```python
from build123d import *

# Parameters (mm, degrees)
SKETCH1_W            = 30
SKETCH1_H            = 70
BOSS_EXTRUDE1_DEPTH  = 1.57
M2_CLEARANCE_HOLE1_D = 2.4
CUT_EXTRUDE1_REACH   = 40.111
SKETCH6_R            = 0.55
LPATTERN1_COUNT      = 15
LPATTERN1_PITCH      = 2.54
SKETCH7_W            = 30
SKETCH7_H            = 20
CUT_EXTRUDE2_DEPTH   = 39.111217509
M2_CLEARANCE_HOLE2_D = 2.4


with BuildPart() as part:
    # Sketch1 → Boss-Extrude1 (new body)
    with BuildSketch(Plane(origin=(0, 0, 0), x_dir=(1, 0, 0), z_dir=(0, 1, 0))):
        Rectangle(SKETCH1_W, SKETCH1_H)
    extrude(amount=BOSS_EXTRUDE1_DEPTH)

    # M2 Clearance Hole1 (through all)
    with Locations(Plane(origin=(0, 1.57, 0), x_dir=(1, 0, 0), z_dir=(0, 1, 0))):
        with Locations((13, 33), (-13, 33), (-13, -33), (13, -33)):
            Hole(M2_CLEARANCE_HOLE1_D / 2)

    # Sketch6 → Cut-Extrude1 (cut, up to next)
    with BuildSketch(Plane(origin=(0, 1.57, 0), x_dir=(1, 0, 0), z_dir=(0, 1, 0)), mode=Mode.PRIVATE) as cut_extrude1_sk1:
        with Locations(Location((6.93, 18.93, 0), (0, 0, 270))):
            Circle(SKETCH6_R)
    cut_extrude1_tool1 = extrude(cut_extrude1_sk1.sketch, amount=-CUT_EXTRUDE1_REACH, mode=Mode.PRIVATE) & part.part
    # Sketch6 → Cut-Extrude1 (cut, up to next)
    with BuildSketch(Plane(origin=(0, 1.57, 0), x_dir=(1, 0, 0), z_dir=(0, 1, 0)), mode=Mode.PRIVATE) as cut_extrude1_sk2:
        with Locations(Location((-8.43, 18.93, 0), (0, 0, 270))):
            Circle(SKETCH6_R)
    cut_extrude1_tool2 = extrude(cut_extrude1_sk2.sketch, amount=-CUT_EXTRUDE1_REACH, mode=Mode.PRIVATE) & part.part
    cut_extrude1_1 = cut_extrude1_tool1.solids().sort_by_distance((6.93, 1.57, -18.93))[0]
    add(cut_extrude1_1, mode=Mode.SUBTRACT)
    cut_extrude1_2 = cut_extrude1_tool2.solids().sort_by_distance((-8.43, 1.57, -18.93))[0]
    add(cut_extrude1_2, mode=Mode.SUBTRACT)
    cut_extrude1 = cut_extrude1_1 + cut_extrude1_2  # Cut-Extrude1 as one shape, for the pattern or mirror that repeats it

    # LPattern1: Cut-Extrude1 ×15
    with Locations(*[(0, 0, i * LPATTERN1_PITCH) for i in range(1, LPATTERN1_COUNT)]):
        add(cut_extrude1, mode=Mode.SUBTRACT)

    # Sketch7 → Cut-Extrude2 (cut, through all)
    with BuildSketch(Plane.XZ):
        with Locations((0, -25)):
            Rectangle(SKETCH7_W, SKETCH7_H)
    extrude(amount=-CUT_EXTRUDE2_DEPTH, mode=Mode.SUBTRACT)

    # M2 Clearance Hole2 (through all)
    with Locations(Plane(origin=(0, 0, 0), x_dir=(-1, 0, 0), z_dir=(0, -1, 0))):
        with Locations((1.4, 3.69)):
            Hole(M2_CLEARANCE_HOLE2_D / 2)


solid = part.part
```
The listing builds one solid part. Answer for the finished solid, in the listing's coordinates (mm). Give positions to 0.01 mm unless a question says otherwise; leave off trailing zeros. Order: outer loops, then holes, each group sorted by start corner. A loop starts at its lowest first (then second) coordinate and runs counter-clockwise, first axis right, second up. Notation, with made-up numbers: (30, -3) -> (84, -3) arc R31 ccw to (84, 30) -> close; hole circle Ø7 at (-20.75, -33). An arc over 180 degrees is marked (long way). One line per item, written item: value.
1) Find the intervals of material crossed by line 1 (X direction, y = 1.05, z = 33); line 2 (X direction, y = 0.15, z = 14); line 3 (X direction, y = 0.55, z = -4), in increasing order.
Reported:
line 1: x = -15 to -14.2, -11.8 to 11.8, 14.2 to 15
line 2: x = -15 to -8.97, -7.89 to 6.39, 7.47 to 15
line 3: x = -15 to -8.88, -7.98 to -2.56, -0.24 to 6.48, 7.38 to 15
2) Determine the mould class of faces 1 (the flat face through (0, 1, -15)), 2 (the cylindrical face through (-7.97, 0.8, -3.39)), 3 (the flat face through (0, 1, 35)) for opening direction Z: pulls with the +Z half, pulls with the -Z half, needs draft (parallel to the pull), parting line crosses it, or undercut.
Reported:
face 1: pulls with the -Z half
face 2: undercut
face 3: pulls with the +Z half
3) Find section B-B, the plane x = 13. Determine the outline of the cut face in (y, z).
Reported:
outline: (0, -15) -> (1.57, -15) -> (1.57, 31.8) -> (0, 31.8) -> close; (0, 34.2) -> (1.57, 34.2) -> (1.57, 35) -> (0, 35) -> close
4) Find section C-C, the plane z = -3.69. Determine the outline of the cut face in (x, y), plus the area to 3 significant figures.
Reported:
outline: (-15, 0) -> (-8.98, 0) -> (-8.98, 1.57) -> (-15, 1.57) -> close; (-7.88, 0) -> (-2.6, 0) -> (-2.6, 1.57) -> (-7.88, 1.57) -> close; (-0.2, 0) -> (6.38, 0) -> (6.38, 1.57) -> (-0.2, 1.57) -> close; (7.48, 0) -> (15, 0) -> (15, 1.57) -> (7.48, 1.57) -> close
area: 39.9 mm^2
5) Find section D-D, the plane y = 0.5. Count the separate pieces of the cut face and the enclosed holes in it, plus the area to 3 significant figures.
Reported:
separate pieces: 1
enclosed holes: 29
area: 1,460 mm^2
6) Find section A-A, the plane z = 6.47. Determine the outline of the cut face in (x, y).
Reported:
outline: (-15, 0) -> (-8.98, 0) -> (-8.98, 1.57) -> (-15, 1.57) -> close; (-7.88, 0) -> (6.38, 0) -> (6.38, 1.57) -> (-7.88, 1.57) -> close; (7.48, 0) -> (15, 0) -> (15, 1.57) -> (7.48, 1.57) -> close
